Geometry check sheet. Reference: the model listing, model coordinates, mm. A direction names the side the tool comes from. Coordinates: 2 decimals unless noted, no trailing zeros. Write each loop counter-clockwise with the first axis right and the second up, starting at its lowest first coordinate (ties: lowest second). Pieces come first, ordered by that corner, then holes. Notation, with made-up numbers: M 69,9.5 L 78,9.5 A29 ccw 78,34.5 Z; hole C -2.75,54 d6. An arc over 180 degrees is marked long. Put each result on its own line as item: value. Start each with the question number.
1) Cross-section at D-D on x = 24. Record the cut outline in (y, z), plus the area to 3 significant figures.
2) Gauge pin test, flat ends, axial feed: pin 1 (2 mm diameter, centred on x = 2, z = -35, fed in from +Y); pin 2 (1.8 mm diameter, centred on x = 51, y = 2, fed in from -Z). Record the tip position at first contact, or that the pin passes through.
3) Set-up check for faces 4 (the cylindrical face through (13.984, 2.133, -38.933)), 5 (the cylindrical face through (62.324, 2.045, -36.024)), 6 (the cylindrical face through (13.984, 2.133, 38.933)), 7 (the flat face through (22.947, 2, -30)): record each of +Z, -Z, +X, -X, +Y, -Y from which the full face is reachable in a straight line by a thin tool's end or side.
4) Cross-section at A-A on x = 33. Record the cut outline in (y, z) (3 decimals), plus the area to 3 significant figures.
5) Cross-section at C-C on x = 2. Record the cut outline in (y, z), plus the area to 3 significant figures.
6) Cross-section at B-B on z = 24.5. Record the cut outline in (x, y).
7) Scan lines: line 1 along Z through (x, y) = (2, 2.8); line 2 along Z through (x, y) = (31.5, 0.5); line 3 along Z through (x, y) = (61.5, 2) (3 decimals). Record each from-to range of solid material in increasing order.
8) Mould release check, pull along Y, two halves, no side actions. Record for faces 1 (the flat face through (44.447, 2, -30)), 2 (the flat face through (33, 0, -1)), 3 (the cylindrical face through (62.32, 1, -0.22)): released by +Y, released by -Y, zero draft, split by the parting line, or undercut.
from build123d import *

# Parameters (mm, degrees)
SKETCH_1_R                    = 1.25
EXTRUDE_1_DEPTH               = 4
SKETCH_2_W                    = 21.5
SKETCH_2_H                    = 20
CUT_EXTRUDE_1_DEPTH           = 8
HOLE_WIZARD_M2_5_1_AT_2_COUNT = 2
HOLE_WIZARD_M2_5_1_AT_2_PITCH = 18
HOLE_WIZARD_M2_5_1_AT_3_COUNT = 2
HOLE_WIZARD_M2_5_1_AT_3_PITCH = 36
HOLE_WIZARD_M2_5_2_D          = 2.05
HOLE_WIZARD_M2_5_2_DEPTH      = 7.25
HOLE_WIZARD_M2_5_2_TIP        = 0.615882135


with BuildPart() as part:
    # 草图1 → 凸台-拉伸1 (new body)
    with BuildSketch(Plane(origin=(0, 0, 0), x_dir=(1, 0, 0), z_dir=(0, 1, 0))):
        Polygon((0, 0), (0, 43), (66, 43), (66, -43), (0, -43), align=None)
        with Locations((2, 0)):
            Circle(SKETCH_1_R, mode=Mode.SUBTRACT)
        with Locations((2, 35)):
            Circle(SKETCH_1_R, mode=Mode.SUBTRACT)
        with Locations((2, -35)):
            Circle(SKETCH_1_R, mode=Mode.SUBTRACT)
    extrude(amount=EXTRUDE_1_DEPTH)

    # 草图2 → 切除-拉伸1 (cut)
    with BuildSketch(Plane(origin=(0, 0, 0), x_dir=(1, 0, 0), z_dir=(0, 1, 0))):
        with Locations((33.697153025, -30)):
            Rectangle(SKETCH_2_W, SKETCH_2_H)
        with Locations((33.697153025, 30)):
            Rectangle(SKETCH_2_W, SKETCH_2_H)
    extrude(amount=CUT_EXTRUDE_1_DEPTH, mode=Mode.SUBTRACT)

    # 草图6 → M2.5 螺纹孔1 (revolve, cut)
    with BuildSketch(Plane(origin=(15, 2, 43), x_dir=(0, -1, 0), z_dir=(1, 0, 0))):
        Polygon((0, 0), (0, 8.865882135), (1.025, 8.25), (1.025, 0), align=None)
    hole_wizard_m2_5_1 = revolve(axis=Axis((15, 2, 49.35), (0, 0, -1)), mode=Mode.SUBTRACT)

    # M2.5 螺纹孔1 at 2: M2.5 螺纹孔1 ×2
    with Locations(*[(i * HOLE_WIZARD_M2_5_1_AT_2_PITCH, 0, 0) for i in range(1, HOLE_WIZARD_M2_5_1_AT_2_COUNT)]):
        add(hole_wizard_m2_5_1, mode=Mode.SUBTRACT)

    # M2.5 螺纹孔1 at 3: M2.5 螺纹孔1 ×2
    with Locations(*[(i * HOLE_WIZARD_M2_5_1_AT_3_PITCH, 0, 0) for i in range(1, HOLE_WIZARD_M2_5_1_AT_3_COUNT)]):
        add(hole_wizard_m2_5_1, mode=Mode.SUBTRACT)

    # 镜向1: M2.5 螺纹孔1 across plane
    add(hole_wizard_m2_5_1.mirror(Plane.XY), mode=Mode.SUBTRACT)

    # 镜向1 copy 1 sketch → 镜向1 copy 1 (revolve, cut)
    with BuildSketch(Plane(origin=(33, 2, -43), x_dir=(0, -1, 0), z_dir=(1, 0, 0))):
        Polygon((0, 0), (0, -8.865882135), (1.025, -8.25), (1.025, 0), align=None)
    revolve(axis=Axis((33, 2, -49.35), (0, 0, -1)), mode=Mode.SUBTRACT)

    # 镜向1 copy 2 sketch → 镜向1 copy 2 (revolve, cut)
    with BuildSketch(Plane(origin=(51, 2, -43), x_dir=(0, -1, 0), z_dir=(1, 0, 0))):
        Polygon((0, 0), (0, -8.865882135), (1.025, -8.25), (1.025, 0), align=None)
    revolve(axis=Axis((51, 2, -49.35), (0, 0, -1)), mode=Mode.SUBTRACT)

    # M2.5 螺纹孔2
    with Locations(Plane(origin=(66, 0, 0), x_dir=(0, 0, -1), z_dir=(1, 0, 0))):
        with Locations((0, 2), (-35, 2), (35, 2)):
            Hole(HOLE_WIZARD_M2_5_2_D / 2, depth=HOLE_WIZARD_M2_5_2_DEPTH)
            with Locations((0, 0, -(HOLE_WIZARD_M2_5_2_DEPTH + HOLE_WIZARD_M2_5_2_TIP / 2))):  # 118° drill point
                Cone(0, HOLE_WIZARD_M2_5_2_D / 2, HOLE_WIZARD_M2_5_2_TIP, mode=Mode.SUBTRACT)


solid = part.part
Answer key:
1. outline: M 0,-43 L 4,-43 L 4,-40 L 0,-40 Z; M 0,-20 L 4,-20 L 4,20 L 0,20 Z; M 0,40 L 4,40 L 4,43 L 0,43 Z
1. area: 184 mm²
2. pin 1: passes through
2. pin 2: stops at z = -34.67
3. face 4: -Z
3. face 5: +X
3. face 6: +Z
3. face 7: +Y, -Y
4. outline: M 0,-43 L 0.975,-43 L 0.975,-40 L 0,-40 Z; M 0,-20 L 4,-20 L 4,20 L 0,20 Z; M 0,40 L 0.975,40 L 0.975,43 L 0,43 Z; M 3.025,-43 L 4,-43 L 4,-40 L 3.025,-40 Z; M 3.025,40 L 4,40 L 4,43 L 3.025,43 Z
4. area: 172 mm²
5. outline: M 0,-43 L 4,-43 L 4,-36.25 L 0,-36.25 Z; M 0,-33.75 L 4,-33.75 L 4,-1.25 L 0,-1.25 Z; M 0,1.25 L 4,1.25 L 4,33.75 L 0,33.75 Z; M 0,36.25 L 4,36.25 L 4,43 L 0,43 Z
5. area: 314 mm²
6. outline: M 0,0 L 22.95,0 L 22.95,4 L 0,4 Z; M 44.45,0 L 66,0 L 66,4 L 44.45,4 Z
7. line 1: z = -43 to -36.25, -33.75 to -1.25, 1.25 to 33.75, 36.25 to 43
7. line 2: z = -43 to -40, -20 to 20, 40 to 43
7. line 3: z = -43 to -36.025, -33.975 to -1.025, 1.025 to 33.975, 36.025 to 43
8. face 1: zero draft
8. face 2: released by -Y
8. face 3: undercut
